Can you work these out from the model? Positions are in its coordinate system, mm. A direction names the side the tool comes from. Give positions to 0.01 mm unless a question says otherwise; leave off trailing zeros. Order: outer loops, then holes, each group sorted by start corner. A loop starts at its lowest first (then second) coordinate and runs counter-clockwise, first axis right, second up. Notation, with made-up numbers: (33.25, 34.5) -> (81.25, 34.5) arc R21 cw to (81.25, 42.5) -> close; hole circle Ø8 at (58.25, 72.5). An arc over 180 degrees is marked (long way). Answer as a JSON object with one key per item and string values.
```python
from build123d import *

# Parameters (mm, degrees)
F1_DEPTH = 63.5
F2_DEPTH = 25.4
F3_DEPTH = 3.175
F0_W     = 41.5249824387
F0_H     = 19.05
F5_R     = 6.35


with BuildPart() as f1:
    # F0 (on Front) → F1 (new body, symmetric)
    with BuildSketch(Plane.XZ):
        Polygon((-41.275, -9.525), (41.275, -9.525), (41.275, 9.525), (22.225, 9.525), (-41.275, 9.525), align=None)
    extrude(amount=F1_DEPTH, both=True)

    # F0 (on Front) → F2 (join, symmetric)
    with BuildSketch(Plane.XZ):
        with BuildLine():
            Line((22.225, 9.525), (41.275, 9.525))
            Line((41.275, 9.525), (41.275, 27.0081188058))
            ThreePointArc((41.275, 27.0081188058), (46.1033585618, 38.409317775), (57.6513575351, 42.8752))
            Line((57.6513575351, 42.8752), (60.325, 42.8752))
            Line((60.325, 42.8752), (60.325, 61.9252))
            Line((60.325, 61.9252), (57.8936839925, 61.9252))
            ThreePointArc((57.8936839925, 61.9252), (53.4742955907, 61.7391542366), (49.1138676774, 60.9960019746))
            ThreePointArc((49.1138676774, 60.9960019746), (29.7600607306, 48.6771485907), (22.225, 27.0081188058))
            Line((22.225, 27.0081188058), (22.225, 9.525))
        make_face()
    extrude(amount=F2_DEPTH, both=True)

    # F0 (on Front) → F3 (join, symmetric)
    with BuildSketch(Plane.XZ):
        with BuildLine():
            add(Edge.make_bspline(
                [(-41.275, 9.525), (-26.5586767346, 33.857088536), (-5.6087374687, 55.4516389966), (49.1138676774, 60.9960019746)],
                knots=[0, 0, 0, 0, 104.0163998813, 104.0163998813, 104.0163998813, 104.0163998813], degree=3))
            Line((-41.275, 9.525), (22.225, 9.525))
            Line((22.225, 9.525), (22.225, 27.0081188058))
            ThreePointArc((22.225, 27.0081188058), (29.7600607306, 48.6771485907), (49.1138676774, 60.9960019746))
        make_face()
    extrude(amount=F3_DEPTH, both=True)

    # F0 (on Front) → F4 (revolve)
    with BuildSketch(Plane.XZ):
        with Locations((81.0874912194, 52.4002)):
            Rectangle(F0_W, F0_H)
    revolve(axis=Axis((60.325, 0, 52.3875), (0, 0, 1)))

    # F5
    f5_edges = [f1.edges().sort_by_distance(p)[0] for p in [
        (41.275, -63.5, 0),
        (-41.275, -63.5, 0),
        (-41.275, 63.5, 0),
        (41.275, 63.5, 0),
    ]]
    fillet(f5_edges, radius=F5_R)


solid = f1.part
```
1. If we section it at A-A on z = -4: Please give me the cut outline in (x, y) (3 decimals).
Worked answers:
{"outline": "(-41.275, -57.15) arc R6.35 ccw to (-34.925, -63.5) -> (34.925, -63.5) arc R6.35 ccw to (41.275, -57.15) -> (41.275, 57.15) arc R6.35 ccw to (34.925, 63.5) -> (-34.925, 63.5) arc R6.35 ccw to (-41.275, 57.15) -> close"}
2. If we section it at C-C on y = 48: Please give me the cut outline in (x, z) (3 decimals).
Worked answers:
{"outline": "(-41.275, -9.525) -> (41.275, -9.525) -> (41.275, 9.525) -> (-41.275, 9.525) -> close"}
3. For faces 4 (the face through (22.225, -14, 18)), 5 (the face through (99.932, 12.473, 52.534)), 6 (the face through (41.275, -1, 4)), which set-ups out of +Z, -Z, +X, -X, +Y, -Y let a thin tool reach every point of the face, with its end or its side?
Worked answers:
{"face 4": "-X, -Y", "face 5": "+Z", "face 6": "-Z, +X, +Y, -Y"}
4. Will these pins go through, and if not, where does the flat tip stop? pin 1 Ø5 at (y, z) = (-18.5, 16) entering from -X (3 decimals); pin 2 Ø12 at (x, z) = (86, 45.5) entering from +Y; pin 3 Ø8 at (x, y) = (-19.5, -2.5) entering from +Z.
Worked answers:
{"pin 1": "x = 22.225", "pin 2": "y = 36.57", "pin 3": "z = 39.21"}
5. If we mould it in two halves opening along Z, with no side actions, what happens to faces 1 (the face through (23, 11, 42.875)), 2 (the face through (61, 1, 61.925)), 3 (the face through (0, 63.5, 0))? For each: +Z half, -Z half, draft (parallel to the pull), parting line (faces both ways), or undercut.
Worked answers:
{"face 1": "undercut", "face 2": "+Z half", "face 3": "draft"}
6. If we section it at B-B on y = 32.5: Please give me the cut outline in (x, z) (3 decimals), then the cut area to 3 significant figures.
Worked answers:
{"outline": "(-41.275, -9.525) -> (41.275, -9.525) -> (41.275, 9.525) -> (-41.275, 9.525) -> close; (34.478, 42.875) -> (86.172, 42.875) -> (86.172, 61.925) -> (34.478, 61.925) -> close", "area": "2,560 mm²"}
7. If we section it at D-D on x = 72: Please give me the cut outline in (y, z).
Worked answers:
{"outline": "(-39.85, 42.88) -> (39.85, 42.88) -> (39.85, 61.93) -> (-39.85, 61.93) -> close"}
8. Please list where these lines run through material, in increasing order: L1, parallel to Z at x = 58.5, y = 6.5; L2, parallel to Z at x = 21, y = 46.5 (3 decimals); L3, parallel to X at y = 24, z = 22.5 (3 decimals).
Worked answers:
{"L1": "42.88 to 61.93", "L2": "-9.525 to 9.525", "L3": "22.225 to 41.275"}
